from build123d import *

# Parameters (mm, degrees)
SKETCH1_W           = 4
SKETCH1_H           = 4
SKETCH1_R           = 1.5
BOSS_EXTRUDE1_DEPTH = 10
SKETCH3_W           = 1.5
SKETCH3_H           = 0.5
BOSS_EXTRUDE2_DEPTH = 1
SKETCH4_W           = 1.5
SKETCH4_H           = 0.5
BOSS_EXTRUDE3_DEPTH = 1


with BuildPart() as part:
    # Sketch1 → Boss-Extrude1 (new body)
    with BuildSketch(Plane.XY):
        Rectangle(SKETCH1_W, SKETCH1_H)
        Circle(SKETCH1_R, mode=Mode.SUBTRACT)
    extrude(amount=BOSS_EXTRUDE1_DEPTH)

    # Sketch3 → Boss-Extrude2 (add)
    with BuildSketch(Plane(origin=(2, 0, 0), x_dir=(0, 0, -1), z_dir=(1, 0, 0))):
        with Locations((-8.75, -1.75)):
            Rectangle(SKETCH3_W, SKETCH3_H)
        with Locations((-1.25, -1.75)):
            Rectangle(SKETCH3_W, SKETCH3_H)
    extrude(amount=BOSS_EXTRUDE2_DEPTH)

    # Sketch4 → Boss-Extrude3 (add)
    with BuildSketch(Plane.ZY.offset(2)):
        with Locations((8.75, -1.75)):
            Rectangle(SKETCH4_W, SKETCH4_H)
    extrude(amount=BOSS_EXTRUDE3_DEPTH)


solid = part.part
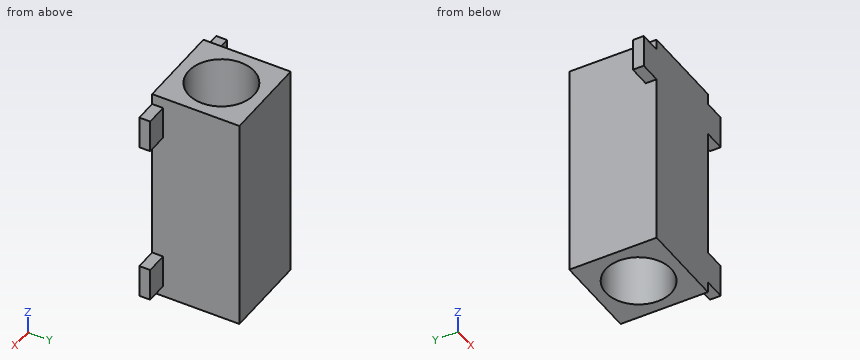
Geometry: final body of the model. Coordinates: model frame, mm. Coordinates: 2 decimals unless noted, no trailing zeros. Loops run counter-clockwise (first coordinate to the right, second up) from the corner with the lowest first, then second, coordinate; pieces in that order, holes last. Notation, with made-up numbers: M 89,-35.75 L 99,-35.75 A29 ccw 99,-1.75 Z; hole C 72,-25.5 d2. An arc over 180 degrees is marked long. One line per item, written item: value. Start each with the question number.
1) Cut plane C-C (x = 0). Return loops of the section in (y, z).
2) Cut plane D-D (z = 1). Return loops of the section in (x, y), then the cut area to 3 significant figures.
3) Pin query (flat end, axial travel): P1, Ø0.6, axis at x = 2.5, y = -1.5, coming from the +Z side; P2, Ø1, axis at x = -0.5, y = 0.5, coming from the +Z side; P3, Ø0.6, axis at x = -2.5, y = -2, coming from the -Z side; P4, Ø0.8, axis at x = 2.5, z = 9, coming from the +Y side. Return the tip coordinate at first contact, or that it passes through.
4) Cut plane A-A (y = -0.9). Return loops of the section in (x, z), then the cut area to 3 significant figures.
5) Cut plane B-B (z = 8.5). Return loops of the section in (x, y), then the cut area to 3 significant figures.
6) Material intervals for L1, parallel to X at y = -0.1, z = 6.75; L2, parallel to X at y = 0.5, z = 9.5, sorted ascending. Write a range as from..to.
Evaluation:
1. outline: M -2,0 L -1.5,0 L -1.5,10 L -2,10 Z; M 1.5,0 L 2,0 L 2,10 L 1.5,10 Z
2. outline: M -2,-2 L 3,-2 L 3,-1.5 L 2,-1.5 L 2,2 L -2,2 Z; hole C 0,0 d3
2. area: 9.43 mm^2
3. P1: z = 9.5
3. P2: through
3. P3: z = 8
3. P4: y = -1.5
4. outline: M -2,0 L -1.2,0 L -1.2,10 L -2,10 Z; M 1.2,0 L 2,0 L 2,10 L 1.2,10 Z
4. area: 16.0 mm^2
5. outline: M -3,-2 L 3,-2 L 3,-1.5 L 2,-1.5 L 2,2 L -2,2 L -2,-1.5 L -3,-1.5 Z; hole C 0,0 d3
5. area: 9.93 mm^2
6. L1: -2..-1.5, 1.5..2
6. L2: -2..-1.41, 1.41..2
